Design review of the part built by this model. Coordinates are the model's own, in mm. A direction names the side the tool comes from. Coordinates: 2 decimals unless noted, no trailing zeros. Loops run counter-clockwise (first coordinate to the right, second up) from the corner with the lowest first, then second, coordinate; pieces in that order, holes last.
from build123d import *

# Parameters (mm, degrees)
EXTRUDE001_DEPTH = 100


with BuildPart() as body002:
    # Sketch → Revolution (revolve)
    with BuildSketch(Plane.XZ):
        with BuildLine():
            Line((0, 0), (0, 135.563389))
            ThreePointArc((23.86226, 121.281178), (13.904936, 131.720055), (0, 135.563389))
            ThreePointArc((32.577943, 87.696618), (30.229669, 105.01041), (23.86226, 121.281178))
            ThreePointArc((22.101567, 52.101534), (30.047255, 69.102202), (32.577943, 87.696618))
            ThreePointArc((22.101567, 52.101534), (13.488015, 26.476163), (18.952965, 0))
            Line((0, 0), (18.952965, 0))
        make_face()
    revolve(axis=Axis((0, 0, 0), (0, 0, 1)))


with BuildPart() as body002_1:
    # Clone001 placement: moved
    add(body002.part.moved(Location((0, -1, 0))))


with BuildPart() as common001:
    # Sketch014 → Extrude001 (new body)
    with BuildSketch(Plane.XZ):
        with BuildLine():
            Line((-19.184126, 99.1166), (-15.572962, 103.201874))
            Line((-15.572962, 103.201874), (-12.116452, 98.911034))
            Line((-12.116452, 98.911034), (-6.872091, 102.963493))
            Line((-6.872091, 102.963493), (0, 98.795265))
            Line((0, 98.795265), (6.11962, 102.844307))
            Line((6.11962, 102.844307), (10.485641, 98.955933))
            Line((10.485641, 98.955933), (14.820494, 102.725113))
            Line((14.820494, 102.725113), (18.947416, 99.223709))
            Line((18.947416, 99.223709), (17.97, 98.527489))
            Line((17.97, 98.527489), (17.97, 86.319122))
            ThreePointArc((-17.97, 86.319122), (0, 68.349122), (17.97, 86.319122))
            Line((-17.97, 98.527489), (-17.97, 86.319122))
            Line((-19.184126, 99.1166), (-17.97, 98.527489))
        make_face()
    extrude(amount=EXTRUDE001_DEPTH)

    # Common001: intersect Body002
    add(body002_1.part, mode=Mode.INTERSECT)


solid = common001.part
Q1. Clearance check with flat-ended pins moving along their axes: pin 1 Ø2 at (x, z) = (-9.5, 96) entering from -Y; pin 2 Ø5 at (x, z) = (6.5, 84) entering from -Y; pin 3 Ø6 at (x, y) = (-13.5, -9) entering from +Z. State where each tip first meets the part, or that it passes through.
Q2. For line 1 (X direction, y = -28, z = 89.5); line 2 (Y direction, x = 4, z = 98); line 3 (Z direction, x = 11, y = -15.5), list the stretches that pass through material, from the lowest coordinate up.
Q3. Machinability: for faces 1 (the flat face through (-17.97, -14, 93)), 2 (the flat face through (3.017, -16.051, 100.791)), 3 (the flat face through (-17.404, -13.522, 101.131)), 4 (the flat face through (17.97, -14, 93)), which of the approach directions +Z, -Z, +X, -X, +Y, -Y give a long, thin tool a straight path to every point of the face, cutting with its end or side? Answer none if there is none.
Q4. Take a section at A-A, the plane y = -3. Write out the cut boundary in (x, z).
Q5. The part is to be moulded in two halves that separate along X. For faces 5 (the flat face through (-18.59, -13.31, 98.83)), 6 (the flat face through (-3.484, -16.051, 100.909)), 7 (the flat face through (16.855, -13.795, 100.999)), say which applies: pulls with the +X half, pulls with the -X half, needs draft (parallel to the pull), parting line crosses it, or undercut.
Q6. Take a section at B-B, the plane z = 100.5. Give the number of separate pieces and of enclosed holes in the cut face, then the cut area to 3 significant figures.
Entries:
1. pin 1: stops at y = -31.86
1. pin 2: stops at y = -33.29
1. pin 3: stops at z = 103.2
2. line 1: x = -17.97 to 17.97
2. line 2: y = -32.44 to 0
2. line 3: z = 72.11 to 99.4
3. face 1: -Z, -X, +Y, -Y
3. face 2: +Z, +Y, -Y
3. face 3: +Z, -X, +Y, -Y
3. face 4: -Z, +X, +Y, -Y
4. outline: (-19.18, 99.12) - (-17.97, 98.53) - (-17.97, 86.32) arc R17.97 ccw to (17.97, 86.32) - (17.97, 98.53) - (18.95, 99.22) - (14.82, 102.73) - (10.49, 98.96) - (6.12, 102.84) - (0, 98.8) - (-6.87, 102.96) - (-12.12, 98.91) - (-15.57, 103.2) - close
5. face 5: pulls with the -X half
5. face 6: undercut
5. face 7: pulls with the +X half
6. separate pieces: 4
6. enclosed holes: 0
6. area: 699 mm2
